from build123d import *

# Parameters (mm, degrees)
SKETCH_1_R      = 1.75
SKETCH_1_W      = 6
SKETCH_1_H      = 4
SKETCH_1_W_2    = 7
EXTRUDE_6_DEPTH = 2


with BuildPart() as part:
    # ｽｹｯﾁ1 → ﾎﾞｽ - 押し出し6 (new body)
    # profile 1 of 3: a face of its own
    with BuildSketch(Plane.XY):
        Polygon((18, 24), (25, 24), (25, 0), (0, 0), (0, 24), (6, 24), (6, 4), (18, 4), align=None)
        with Locations((23, 9.5)):
            Circle(SKETCH_1_R, mode=Mode.SUBTRACT)
        with Locations((2, 9.5)):
            Circle(SKETCH_1_R, mode=Mode.SUBTRACT)
        with Locations((23, 22)):
            Circle(SKETCH_1_R, mode=Mode.SUBTRACT)
        with Locations((2, 22)):
            Circle(SKETCH_1_R, mode=Mode.SUBTRACT)
    # profile 2 of 3: a face of its own
    with BuildSketch(Plane.XY):
        with Locations((3, 26)):
            Rectangle(SKETCH_1_W, SKETCH_1_H)
    # profile 3 of 3: a face of its own
    with BuildSketch(Plane.XY):
        with Locations((21.5, 26)):
            Rectangle(SKETCH_1_W_2, SKETCH_1_H)
    extrude(amount=EXTRUDE_6_DEPTH)


solid = part.part
Can you work these out from the model? Positions are in its coordinate system, mm. A direction names the side the tool comes from. Round coordinates to 2 decimals unless told otherwise and drop trailing zeros. Write each loop counter-clockwise with the first axis right and the second up, starting at its lowest first coordinate (ties: lowest second). Pieces come first, ordered by that corner, then holes. Notation, with made-up numbers: M 87.5,24.25 L 105.5,24.25 A13 ccw 105.5,41.25 Z; hole C 16,83.25 d3. An arc over 180 degrees is marked long. Use a Markdown table: item, result.
Item 1: For pin 1 Ø3 at (x, y) = (2, 9.5) entering from -Z, with a flat end and sliding along its axis, tell me the tip position at first contact or that it passes through.
Found:
| item | result |
|---|---|
| pin 1 | passes through |
Item 2: Which directions (+Z, -Z, +X, -X, +Y, -Y) give clear straight access to the entire face, cutting with the end or side of a thin tool? Please do faces 1 (the face through (12, 4, 1)), 2 (the face through (25, 14, 1)).
Found:
| item | result |
|---|---|
| face 1 | +Z, -Z, +Y |
| face 2 | +Z, -Z, +X, +Y, -Y |
Item 3: I want a section at A-A (y = 24.5). List the corners of the cut face in (x, z) for me, and give its area (3 significant figures).
Found:
| item | result |
|---|---|
| outline | M 0,0 L 6,0 L 6,2 L 0,2 Z; M 18,0 L 25,0 L 25,2 L 18,2 Z |
| area | 26.0 mm2 |
Item 4: We'd pull the mould along Y, two halves only. Please class faces 3 (the face through (18, 16, 1)), 4 (the face through (1.772, 23.735, 0.986)), 5 (the face through (3, 28, 1)), 6 (the face through (13, 0, 1)): released by +Y, released by -Y, zero draft, split by the parting line, or undercut.
Found:
| item | result |
|---|---|
| face 3 | zero draft |
| face 4 | undercut |
| face 5 | released by +Y |
| face 6 | released by -Y |
Item 5: If I drill on line 1 along Y through (x, z) = (2, 0.75); line 2 along X through (y, z) = (4.75, 1.45); line 3 along X through (y, z) = (21, 0.6), over which ranges is the centre line in solid material (lowest first)? Write a range as [from, to].
Found:
| item | result |
|---|---|
| line 1 | y = [0, 7.75], [11.25, 20.25], [23.75, 28] |
| line 2 | x = [0, 6], [18, 25] |
| line 3 | x = [0, 0.56], [3.44, 6], [18, 21.56], [24.44, 25] |
Item 6: I want a section at C-C (y = 9.5). List the corners of the cut face in (x, z) for me.
Found:
| item | result |
|---|---|
| outline | M 0,0 L 0.25,0 L 0.25,2 L 0,2 Z; M 3.75,0 L 6,0 L 6,2 L 3.75,2 Z; M 18,0 L 21.25,0 L 21.25,2 L 18,2 Z; M 24.75,0 L 25,0 L 25,2 L 24.75,2 Z |
Item 7: I want a section at B-B (x = 23). List the corners of the cut face in (y, z) for me.
Found:
| item | result |
|---|---|
| outline | M 0,0 L 7.75,0 L 7.75,2 L 0,2 Z; M 11.25,0 L 20.25,0 L 20.25,2 L 11.25,2 Z; M 23.75,0 L 28,0 L 28,2 L 23.75,2 Z |
Item 8: I want a section at D-D (z = 0.5). List the corners of the cut face in (x, y) for me.
Found:
| item | result |
|---|---|
| outline | M 0,0 L 25,0 L 25,28 L 18,28 L 18,4 L 6,4 L 6,28 L 0,28 Z; hole C 2,9.5 d3.5; hole C 2,22 d3.5; hole C 23,9.5 d3.5; hole C 23,22 d3.5 |
